from build123d import *


with BuildPart() as part:
    # Sketch1 → Revolve1 (revolve)
    with BuildSketch(Plane.XY, mode=Mode.PRIVATE) as revolve1_sk:
        Polygon((-0.431630681, 32.7), (-2.131630681, 31.68), (-2.131630681, 30.54), (-0.431630681, 29.52), (-2.131630681, 28.5), (-2.131630681, 27.36), (-0.431630681, 26.34), (-2.131630681, 25.32), (-2.131630681, 24.18), (-0.431630681, 23.16), (-2.131630681, 22.14), (-2.131630681, 21), (-0.431630681, 19.98), (-2.131630681, 18.96), (-2.131630681, 17.82), (-0.431630681, 16.8), (-2.131630681, 15.78), (-2.131630681, 14.64), (-0.431630681, 13.62), (-2.131630681, 12.6), (-2.131630681, 11.46), (-0.431630681, 10.44), (-2.131630681, 9.42), (-2.131630681, 8.28), (-0.431630681, 7.26), (-0.431630681, 0), (-0.431630681, -0.8), (-5.431630681, -0.8), (-5.431630681, 0), (-1.231630681, 0), (-1.231630681, 6.795995819), (-1.995791511, 7.26), (-3.138866015, 7.96), (-3.138866015, 9.754155298), (-1.995791511, 10.44), (-3.138866015, 11.14), (-3.138866015, 12.934155298), (-1.995791511, 13.62), (-3.138866015, 14.32), (-3.138866015, 16.114155298), (-1.995791511, 16.8), (-3.138866015, 17.5), (-3.138866015, 19.294155298), (-1.995791511, 19.98), (-3.138866015, 20.68), (-3.138866015, 22.474155298), (-1.995791511, 23.16), (-3.138866015, 23.86), (-3.138866015, 25.654155298), (-1.995791511, 26.34), (-3.138866015, 27.04), (-3.138866015, 28.834155298), (-1.995791511, 29.52), (-3.138866015, 30.22), (-3.138866015, 32.014155298), (-1.995791511, 32.7), (-3.138866015, 33.4), (-5.431630681, 33.4), (-5.431630681, 34.2), (-2.931630681, 34.2), align=None)
    revolve(revolve1_sk.sketch.rotate(Axis((-5.431630681, 34.2, 0), (0, -1, 0)), 180), axis=Axis((-5.431630681, 34.2, 0), (0, -1, 0)))


solid = part.part
Part model, mm, in its own coordinate system. A direction names the side the tool comes from. Coordinates: 2 decimals unless noted, no trailing zeros. Order: outer loops, then holes, each group sorted by start corner. A loop starts at its lowest first (then second) coordinate and runs counter-clockwise, first axis right, second up.
(1) Tool access for faces 4 (the face through (-3.14, 21.59, -0.1)), 5 (the face through (-5, 34.2, 0)): list every direction of +Z, -Z, +X, -X, +Y, -Y with a clear straight run to the whole face (end or side of a thin tool).
Check sheet entries:
face 4: none
face 5: +Z, -Z, +X, -X, +Y
(2) Pull direction X, two halves, no side cores. Call faces 1 (the face through (-5, -0.8, 0)), 2 (the face through (-3.14, 18.41, -0.1)), 3 (the face through (-7.965, 34.106, -0.798)): pulls with the +X half, pulls with the -X half, needs draft (parallel to the pull), parting line crosses it, or undercut.
Check sheet entries:
face 1: needs draft
face 2: undercut
face 3: parting line crosses it
(3) Slice it at A-A, the plane y = 9. Write the cut outline in (x, z), and give its area (3 significant figures).
Check sheet entries:
outline: circle Ø6.6 at (-5.43, 0); hole circle Ø4.59 at (-5.43, 0)
area: 17.7 mm2
(4) Pin check, flat tips, straight feed: pin 1 Ø1 at (y, z) = (10.5, 2) entering from -X; pin 2 Ø3 at (y, z) = (21, -3) entering from -X; pin 3 Ø1 at (x, y) = (-9, 29.5) entering from +Z. Stop position of each tip, or through.
Check sheet entries:
pin 1: stops at x = -10.2
pin 2: stops at x = -10.06
pin 3: stops at z = 3.95
(5) Probe L1, parallel to Y at x = -4, z = 0; L2, parallel to Z at x = -6, y = 11.5; L3, parallel to Z at x = -6.5, y = 17. List the from-to ranges inside material, lowest first.
Check sheet entries:
L1: y = -0.8 to 0, 33.4 to 34.2
L2: z = -3.25 to -2.22, 2.22 to 3.25
L3: z = -4.54 to -2.92, 2.92 to 4.54
